For this review, use the dimensioned drawing (mm, ordinates from the lowest corner) and the shaded views. A direction names the side the tool comes from. Coordinates: 2 decimals unless noted, no trailing zeros. Write each loop counter-clockwise with the first axis right and the second up, starting at its lowest first coordinate (ties: lowest second). Pieces come first, ordered by that corner, then holes.
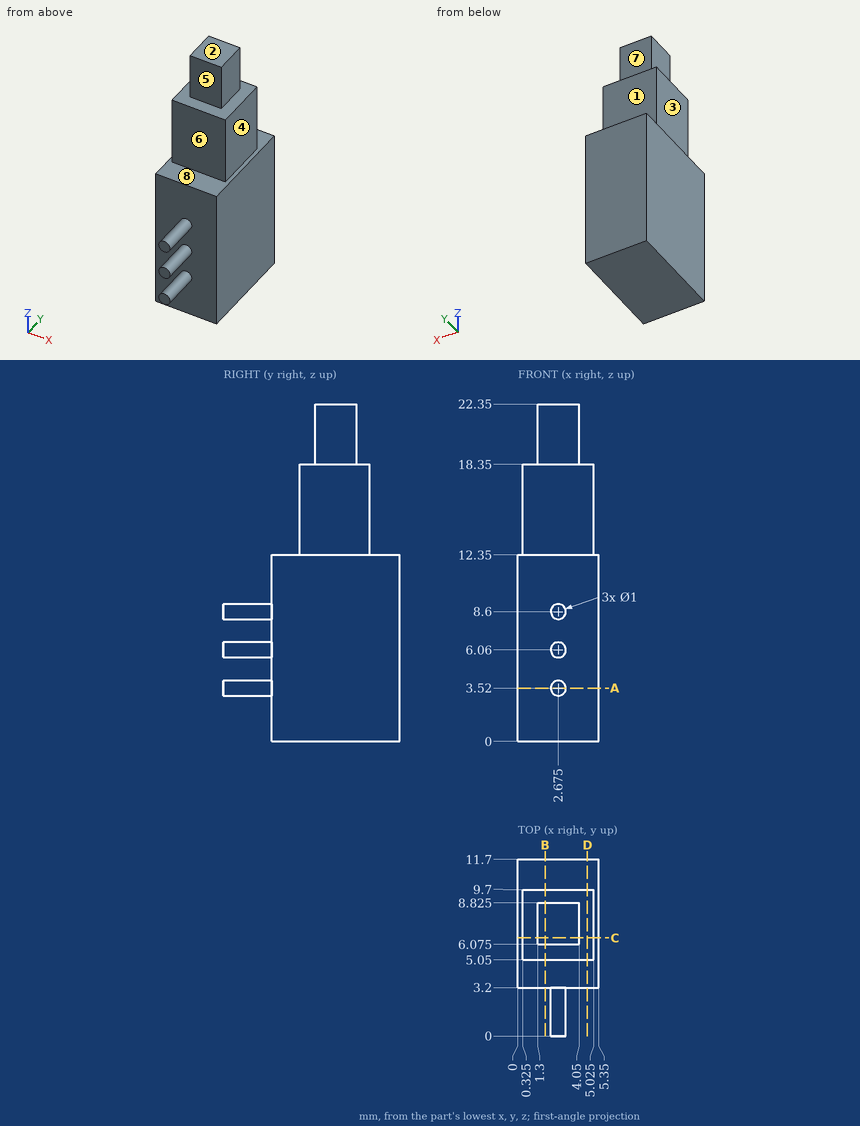
Item 1: To check wall thickness, follow line 1 along Z through (x, y) = (2.2, 4); line 2 along Y through (x, z) = (0.9, 9); line 3 along Z through (x, y) = (4.9, 6.5). State the ranges of each line that lie inside material, in increasing order.
Solved:
line 1: z = 0 to 12.35
line 2: y = 3.2 to 11.7
line 3: z = 0 to 18.35
Item 2: Take a section at C-C, the plane y = 6.5. Write out the cut boundary in (x, z) (3 decimals), plus the area to 3 significant figures.
Solved:
outline: (0, 0) - (5.35, 0) - (5.35, 12.35) - (5.025, 12.35) - (5.025, 18.35) - (4.05, 18.35) - (4.05, 22.35) - (1.3, 22.35) - (1.3, 18.35) - (0.325, 18.35) - (0.325, 12.35) - (0, 12.35) - close
area: 105 mm2
Item 3: Take a section at D-D, the plane x = 4.6. Write out the cut boundary in (y, z).
Solved:
outline: (3.2, 0) - (11.7, 0) - (11.7, 12.35) - (9.7, 12.35) - (9.7, 18.35) - (5.05, 18.35) - (5.05, 12.35) - (3.2, 12.35) - close
Item 4: Machinability: for the marked faces 1, 2, 3, 4 and 5, which of the approach directions +Z, -Z, +X, -X, +Y, -Y give a long, thin tool a straight path to every point of the face, cutting with its end or side? Answer none if there is none.
Solved:
face 1: +Z, +X, -X, +Y
face 2: +Z, +X, -X, +Y, -Y
face 3: +Z, -X, +Y, -Y
face 4: +Z, +X, +Y, -Y
face 5: +Z, +X, -X, -Y
Item 5: Take a section at A-A, the plane z = 3.52. Write out the cut boundary in (x, y) (3 decimals).
Solved:
outline: (0, 3.2) - (2.175, 3.2) - (2.175, 0) - (3.175, 0) - (3.175, 3.2) - (5.35, 3.2) - (5.35, 11.7) - (0, 11.7) - close
Item 6: Mouldability with a two-part tool opening along Y and no side actions: class the marked faces 6, 7 and 8 as pulls with the +Y half, pulls with the -Y half, needs draft (parallel to the pull), parting line crosses it, or undercut.
Solved:
face 6: pulls with the -Y half
face 7: pulls with the +Y half
face 8: needs draft
Item 7: For pin 1 (3 mm diameter, centred on x = 2.5, z = 19.5, fed in from +Y); pin 2 (1.5 mm diameter, centred on x = 2.5, y = 10, fed in from +Z); pin 3 (1.5 mm diameter, centred on y = 3.5, z = 15.5, fed in from -X); pin 4 (2 mm diameter, centred on y = 7, z = 19.5, fed in from +X), all flat-tipped, find the tip position at first contact; note any pin that passes through.
Solved:
pin 1: stops at y = 9.7
pin 2: stops at z = 18.35
pin 3: passes through
pin 4: stops at x = 4.05
Item 8: Take a section at B-B, the plane x = 1.8. Write out the cut boundary in (y, z) (3 decimals), plus the area to 3 significant figures.
Solved:
outline: (3.2, 0) - (11.7, 0) - (11.7, 12.35) - (9.7, 12.35) - (9.7, 18.35) - (8.825, 18.35) - (8.825, 22.35) - (6.075, 22.35) - (6.075, 18.35) - (5.05, 18.35) - (5.05, 12.35) - (3.2, 12.35) - close
area: 144 mm2
